Model file for the job. Use its own axes, mm. A direction names the side the tool comes from. Give positions to 0.01 mm unless a question says otherwise; leave off trailing zeros. Order: outer loops, then holes, each group sorted by start corner. A loop starts at its lowest first (then second) coordinate and runs counter-clockwise, first axis right, second up. Notation, with made-up numbers: (87, 26) - (91, 26) arc R29 ccw to (91, 46) - close; hole circle Ø5 at (-28.5, -17). An arc over 180 degrees is marked (long way). Use CSV: the item, a comma, the result in double quotes. Start each with the question number.
(1) Band-saw the part on B-B, the plane x = 39.5. Give the cut face in (y, z), then the cut area to 3 significant figures.
(2) Probe L1, parallel to Z at x = 31.75, y = 4; L2, parallel to Z at x = -19.05, y = 6; L3, parallel to X at y = 6.5, z = 4. List the from-to ranges inside material, lowest first.
(3) Band-saw the part on D-D, the plane x = 0. Give the cut face in (y, z).
(4) Band-saw the part on C-C, the plane y = 5.5. Count the separate pieces of the cut face and the enclosed holes in it, then the cut area to 3 significant figures.
(5) Drop flat-ended pins along their axis: pin 1 Ø4 at (x, y) = (-21, 5.5) entering from +Z; pin 2 Ø2.5 at (x, y) = (10.5, 5.5) entering from -Z; pin 3 Ø17.5 at (x, z) = (31.75, 0) entering from -Y; pin 4 Ø4 at (y, z) = (6, -11) entering from +X. Give the stop position or say it passes through.
(6) Pull direction Z, two halves, no side cores. Call faces 3 (the cylindrical face through (-28.196, 3.757, -2.88)), 4 (the flat face through (8, 7.62, 0)), 5 (the flat face through (2, 4, 14.288)): +Z half, -Z half, draft (parallel to the pull), parting line (faces both ways), or undercut.
(7) Tool access for faces 1 (the cylindrical face through (21.532, 3.757, 4.237)), 2 (the flat face through (2, 4, -14.288)): list every direction of +Z, -Z, +X, -X, +Y, -Y with a clear straight run to the whole face (end or side of a thin tool).
(8) Band-saw the part on A-A, the plane z = 0. Give the cut face in (x, y), then the cut area to 3 significant figures.
Autodesk Inventor part; units mm, degrees
ref_plane "YZ Plane" through (0, 0, 0) normal (1, 0, 0) x (0, 1, 0)
ref_plane "XZ Plane" through (0, 0, 0) normal (0, 1, 0) x (-1, 0, 0)
ref_plane "XY Plane" through (0, 0, 0) normal (0, 0, 1) x (1, 0, 0)
sketch "Sketch1" plane through (0, 0, 0) normal (0, 1, 0) x (-1, 0, 0)
  arc A0 (-23.4767, 14.2875) -> (-23.4767, -14.2875) centre (-31.75, 0) ccw
  circle A1 centre (-31.75, 0) radius 11.0617
  circle A2 centre (19.05, 0) radius 9.5885
  arc A3 (19.05, -14.2875) -> (19.05, 14.2875) centre (19.05, 0) ccw
  line L0 (19.05, -14.2875) -> (-23.4767, -14.2875)
  line L1 (19.05, 14.2875) -> (-23.4767, 14.2875)
  point P0 (0, 0)
  point P1 (12.5046, 12.7)
  point P2 (-21.2006, -12.7)
  dimension "d11" = 19.177
  dimension "d14" = 28.575
  dimension "d15" = 22.1234
extrude "Extrusion1" add sketch "Sketch1" along normal blind 7.62
properties part number "Connecting Rod"
Answer block:
1,outline,"(0, -14.58) - (7.62, -14.58) - (7.62, -7.89) - (0, -7.89) - close; (0, 7.89) - (7.62, 7.89) - (7.62, 14.58) - (0, 14.58) - close"
1,area,"102 mm2"
2,L1,"z = -16.51 to -11.06, 11.06 to 16.51"
2,L2,"z = -14.29 to -9.59, 9.59 to 14.29"
2,L3,"x = -32.77 to -27.76, -10.34 to 21.44, 42.06 to 47.77"
3,outline,"(0, -14.29) - (7.62, -14.29) - (7.62, 14.29) - (0, 14.29) - close"
4,separate pieces,"1"
4,enclosed holes,"2"
4,area,"1,550 mm2"
5,pin 1,"stops at z = 14.29"
5,pin 2,"stops at z = -14.29"
5,pin 3,"passes through"
5,pin 4,"stops at x = 45.59"
6,face 3,"undercut"
6,face 4,"draft"
6,face 5,"+Z half"
7,face 1,"+Y, -Y"
7,face 2,"-Z, -X, +Y, -Y"
8,outline,"(-33.34, 0) - (-28.64, 0) - (-28.64, 7.62) - (-33.34, 7.62) - close; (-9.46, 0) - (20.69, 0) - (20.69, 7.62) - (-9.46, 7.62) - close; (42.81, 0) - (48.26, 0) - (48.26, 7.62) - (42.81, 7.62) - close"
8,area,"307 mm2"
